```python
from build123d import *

# Parameters (mm, degrees)
SKETCH1_W                    = 31.75
SKETCH1_H                    = 63.5
SKETCH1_W_2                  = 25.4
SKETCH1_H_2                  = 57.15
BOSS_EXTRUDE1_DEPTH          = 685.8
CUT_EXTRUDE1_REACH           = 691.238
SKETCH3_W                    = 50.8
SKETCH3_H                    = 25.4
F_10_0_1935_DIAMETER_HOLE1_D = 4.9149
CUT_EXTRUDE2_REACH           = 691.238
SKETCH6_R                    = 15.5575
SKETCH6_R_2                  = 3.175
CUT_EXTRUDE3_REACH           = 691.238
SKETCH7_R                    = 6.35


with BuildPart() as part:
    # Sketch1 → Boss-Extrude1 (new body)
    with BuildSketch(Plane.XY):
        with Locations((3.710272719, -29.23968021)):
            Rectangle(SKETCH1_W, SKETCH1_H)
        with Locations((3.710272719, -29.23968021)):
            Rectangle(SKETCH1_W_2, SKETCH1_H_2, mode=Mode.SUBTRACT)
    extrude(amount=BOSS_EXTRUDE1_DEPTH)

    # Cut-Extrude1: up to this face of the body (flat: up to its plane)
    cut_extrude1_end = Plane(part.part.faces().sort_by_distance((19.585272719, -29.23968021, 342.9))[0])
    # Sketch3 → Cut-Extrude1 (cut, up to the picked face)
    with BuildSketch(Plane.ZY.offset(12.164727281), mode=Mode.PRIVATE) as cut_extrude1_sk1:
        with BuildLine():
            Line((31.7754, -13.36468021), (120.6754, -13.36468021))
            ThreePointArc((120.6754, -13.36468021), (122.92046403, -14.294616179), (123.8504, -16.53968021))
            Line((123.8504, -16.53968021), (123.8504, -41.93968021))
            ThreePointArc((123.8504, -41.93968021), (122.92046403, -44.18474424), (120.6754, -45.11468021))
            Line((120.6754, -45.11468021), (31.7754, -45.11468021))
            ThreePointArc((31.7754, -45.11468021), (29.53033597, -44.18474424), (28.6004, -41.93968021))
            Line((28.6004, -41.93968021), (28.6004, -16.53968021))
            ThreePointArc((28.6004, -16.53968021), (29.53033597, -14.294616179), (31.7754, -13.36468021))
        make_face()
    cut_extrude1_tool1 = split(extrude(cut_extrude1_sk1.sketch, amount=-CUT_EXTRUDE1_REACH, mode=Mode.PRIVATE), bisect_by=cut_extrude1_end, keep=Keep.BOTH, mode=Mode.PRIVATE)
    # Sketch3 → Cut-Extrude1 (cut, up to the picked face)
    with BuildSketch(Plane.ZY.offset(12.164727281), mode=Mode.PRIVATE) as cut_extrude1_sk2:
        with BuildLine():
            ThreePointArc((657.1996, -41.93968021), (656.26966403, -44.18474424), (654.0246, -45.11468021))
            Line((654.0246, -45.11468021), (565.1246, -45.11468021))
            ThreePointArc((565.1246, -45.11468021), (562.87953597, -44.18474424), (561.9496, -41.93968021))
            Line((561.9496, -41.93968021), (561.9496, -16.53968021))
            ThreePointArc((561.9496, -16.53968021), (562.87953597, -14.294616179), (565.1246, -13.36468021))
            Line((565.1246, -13.36468021), (654.0246, -13.36468021))
            ThreePointArc((654.0246, -13.36468021), (656.26966403, -14.294616179), (657.1996, -16.53968021))
            Line((657.1996, -16.53968021), (657.1996, -41.93968021))
        make_face()
    cut_extrude1_tool2 = split(extrude(cut_extrude1_sk2.sketch, amount=-CUT_EXTRUDE1_REACH, mode=Mode.PRIVATE), bisect_by=cut_extrude1_end, keep=Keep.BOTH, mode=Mode.PRIVATE)
    # Sketch3 → Cut-Extrude1 (cut, up to the picked face)
    with BuildSketch(Plane.ZY.offset(12.164727281), mode=Mode.PRIVATE) as cut_extrude1_sk3:
        with Locations((215.9, -48.28968021)):
            Rectangle(SKETCH3_W, SKETCH3_H)
    cut_extrude1_tool3 = split(extrude(cut_extrude1_sk3.sketch, amount=-CUT_EXTRUDE1_REACH, mode=Mode.PRIVATE), bisect_by=cut_extrude1_end, keep=Keep.BOTH, mode=Mode.PRIVATE)
    # Sketch3 → Cut-Extrude1 (cut, up to the picked face)
    with BuildSketch(Plane.ZY.offset(12.164727281), mode=Mode.PRIVATE) as cut_extrude1_sk4:
        with Locations((469.9, -48.28968021)):
            Rectangle(SKETCH3_W, SKETCH3_H)
    cut_extrude1_tool4 = split(extrude(cut_extrude1_sk4.sketch, amount=-CUT_EXTRUDE1_REACH, mode=Mode.PRIVATE), bisect_by=cut_extrude1_end, keep=Keep.BOTH, mode=Mode.PRIVATE)
    add(cut_extrude1_tool1.solids().sort_by(Axis((-12.164727, -29.23968, 76.2254), (1, 0, 0)))[0], mode=Mode.SUBTRACT)
    add(cut_extrude1_tool2.solids().sort_by(Axis((-12.164727, -29.23968, 609.5746), (1, 0, 0)))[0], mode=Mode.SUBTRACT)
    add(cut_extrude1_tool3.solids().sort_by(Axis((-12.164727, -48.28968, 215.9), (1, 0, 0)))[0], mode=Mode.SUBTRACT)
    add(cut_extrude1_tool4.solids().sort_by(Axis((-12.164727, -48.28968, 469.9), (1, 0, 0)))[0], mode=Mode.SUBTRACT)

    # #10 (0.1935) Diameter Hole1 (through all)
    with Locations(Plane(origin=(3.710272719, 2.51031979, 677.8625), x_dir=(1, 0, 0), z_dir=(0, 1, 0))):
        with Locations((0, 0), (0, 669.925)):
            Hole(F_10_0_1935_DIAMETER_HOLE1_D / 2)

    # Cut-Extrude2: up to this face of the body (flat: up to its plane)
    cut_extrude2_end = Plane(part.part.faces().sort_by_distance((-12.164727281, -27.832525424, 342.9))[0])
    # Sketch6 → Cut-Extrude2 (cut, up to the picked face)
    with BuildSketch(Plane(origin=(19.585272719, 0, 0), x_dir=(0, 0, -1), z_dir=(1, 0, 0)), mode=Mode.PRIVATE) as cut_extrude2_sk1:
        with Locations(Location((-342.9, -34.00218021, 0), (0, 0, 90))):
            Circle(SKETCH6_R)
    cut_extrude2_tool1 = split(extrude(cut_extrude2_sk1.sketch, amount=-CUT_EXTRUDE2_REACH, mode=Mode.PRIVATE), bisect_by=cut_extrude2_end, keep=Keep.BOTH, mode=Mode.PRIVATE)
    # Sketch6 → Cut-Extrude2 (cut, up to the picked face)
    with BuildSketch(Plane(origin=(19.585272719, 0, 0), x_dir=(0, 0, -1), z_dir=(1, 0, 0)), mode=Mode.PRIVATE) as cut_extrude2_sk2:
        with Locations(Location((-393.7, -34.00218021, 0), (0, 0, 90))):
            Circle(SKETCH6_R)
    cut_extrude2_tool2 = split(extrude(cut_extrude2_sk2.sketch, amount=-CUT_EXTRUDE2_REACH, mode=Mode.PRIVATE), bisect_by=cut_extrude2_end, keep=Keep.BOTH, mode=Mode.PRIVATE)
    # Sketch6 → Cut-Extrude2 (cut, up to the picked face)
    with BuildSketch(Plane(origin=(19.585272719, 0, 0), x_dir=(0, 0, -1), z_dir=(1, 0, 0)), mode=Mode.PRIVATE) as cut_extrude2_sk3:
        with Locations(Location((-434.975, -7.01468021, 0), (0, 0, 90))):
            Circle(SKETCH6_R_2)
    cut_extrude2_tool3 = split(extrude(cut_extrude2_sk3.sketch, amount=-CUT_EXTRUDE2_REACH, mode=Mode.PRIVATE), bisect_by=cut_extrude2_end, keep=Keep.BOTH, mode=Mode.PRIVATE)
    # Sketch6 → Cut-Extrude2 (cut, up to the picked face)
    with BuildSketch(Plane(origin=(19.585272719, 0, 0), x_dir=(0, 0, -1), z_dir=(1, 0, 0)), mode=Mode.PRIVATE) as cut_extrude2_sk4:
        with Locations(Location((-301.625, -7.01468021, 0), (0, 0, 90))):
            Circle(SKETCH6_R_2)
    cut_extrude2_tool4 = split(extrude(cut_extrude2_sk4.sketch, amount=-CUT_EXTRUDE2_REACH, mode=Mode.PRIVATE), bisect_by=cut_extrude2_end, keep=Keep.BOTH, mode=Mode.PRIVATE)
    # Sketch6 → Cut-Extrude2 (cut, up to the picked face)
    with BuildSketch(Plane(origin=(19.585272719, 0, 0), x_dir=(0, 0, -1), z_dir=(1, 0, 0)), mode=Mode.PRIVATE) as cut_extrude2_sk5:
        with Locations(Location((-434.975, -51.46468021, 0), (0, 0, 90))):
            Circle(SKETCH6_R_2)
    cut_extrude2_tool5 = split(extrude(cut_extrude2_sk5.sketch, amount=-CUT_EXTRUDE2_REACH, mode=Mode.PRIVATE), bisect_by=cut_extrude2_end, keep=Keep.BOTH, mode=Mode.PRIVATE)
    # Sketch6 → Cut-Extrude2 (cut, up to the picked face)
    with BuildSketch(Plane(origin=(19.585272719, 0, 0), x_dir=(0, 0, -1), z_dir=(1, 0, 0)), mode=Mode.PRIVATE) as cut_extrude2_sk6:
        with Locations(Location((-301.625, -51.46468021, 0), (0, 0, 90))):
            Circle(SKETCH6_R_2)
    cut_extrude2_tool6 = split(extrude(cut_extrude2_sk6.sketch, amount=-CUT_EXTRUDE2_REACH, mode=Mode.PRIVATE), bisect_by=cut_extrude2_end, keep=Keep.BOTH, mode=Mode.PRIVATE)
    add(cut_extrude2_tool1.solids().sort_by(Axis((19.585273, -34.00218, 342.9), (-1, 0, 0)))[0], mode=Mode.SUBTRACT)
    add(cut_extrude2_tool2.solids().sort_by(Axis((19.585273, -34.00218, 393.7), (-1, 0, 0)))[0], mode=Mode.SUBTRACT)
    add(cut_extrude2_tool3.solids().sort_by(Axis((19.585273, -7.01468, 434.975), (-1, 0, 0)))[0], mode=Mode.SUBTRACT)
    add(cut_extrude2_tool4.solids().sort_by(Axis((19.585273, -7.01468, 301.625), (-1, 0, 0)))[0], mode=Mode.SUBTRACT)
    add(cut_extrude2_tool5.solids().sort_by(Axis((19.585273, -51.46468, 434.975), (-1, 0, 0)))[0], mode=Mode.SUBTRACT)
    add(cut_extrude2_tool6.solids().sort_by(Axis((19.585273, -51.46468, 301.625), (-1, 0, 0)))[0], mode=Mode.SUBTRACT)

    # Sketch7 → Cut-Extrude3 (cut, up to next)
    with BuildSketch(Plane(origin=(19.585272719, 0, 0), x_dir=(0, 0, -1), z_dir=(1, 0, 0)), mode=Mode.PRIVATE) as cut_extrude3_sk1:
        with Locations(Location((-434.975, -7.01468021, 0), (0, 0, 90))):
            Circle(SKETCH7_R)
    cut_extrude3_tool1 = extrude(cut_extrude3_sk1.sketch, amount=-CUT_EXTRUDE3_REACH, mode=Mode.PRIVATE) & part.part
    # Sketch7 → Cut-Extrude3 (cut, up to next)
    with BuildSketch(Plane(origin=(19.585272719, 0, 0), x_dir=(0, 0, -1), z_dir=(1, 0, 0)), mode=Mode.PRIVATE) as cut_extrude3_sk2:
        with Locations(Location((-434.975, -51.46468021, 0), (0, 0, 90))):
            Circle(SKETCH7_R)
    cut_extrude3_tool2 = extrude(cut_extrude3_sk2.sketch, amount=-CUT_EXTRUDE3_REACH, mode=Mode.PRIVATE) & part.part
    # Sketch7 → Cut-Extrude3 (cut, up to next)
    with BuildSketch(Plane(origin=(19.585272719, 0, 0), x_dir=(0, 0, -1), z_dir=(1, 0, 0)), mode=Mode.PRIVATE) as cut_extrude3_sk3:
        with Locations(Location((-301.625, -51.46468021, 0), (0, 0, 90))):
            Circle(SKETCH7_R)
    cut_extrude3_tool3 = extrude(cut_extrude3_sk3.sketch, amount=-CUT_EXTRUDE3_REACH, mode=Mode.PRIVATE) & part.part
    # Sketch7 → Cut-Extrude3 (cut, up to next)
    with BuildSketch(Plane(origin=(19.585272719, 0, 0), x_dir=(0, 0, -1), z_dir=(1, 0, 0)), mode=Mode.PRIVATE) as cut_extrude3_sk4:
        with Locations(Location((-301.625, -7.01468021, 0), (0, 0, 90))):
            Circle(SKETCH7_R)
    cut_extrude3_tool4 = extrude(cut_extrude3_sk4.sketch, amount=-CUT_EXTRUDE3_REACH, mode=Mode.PRIVATE) & part.part
    add(cut_extrude3_tool1.solids().sort_by_distance((19.585273, -7.01468, 434.975))[0], mode=Mode.SUBTRACT)
    add(cut_extrude3_tool2.solids().sort_by_distance((19.585273, -51.46468, 434.975))[0], mode=Mode.SUBTRACT)
    add(cut_extrude3_tool3.solids().sort_by_distance((19.585273, -51.46468, 301.625))[0], mode=Mode.SUBTRACT)
    add(cut_extrude3_tool4.solids().sort_by_distance((19.585273, -7.01468, 301.625))[0], mode=Mode.SUBTRACT)


solid = part.part
```
Input: part model. Units: mm. Frame: model coordinates. A direction names the side the tool comes from. Round coordinates to 2 decimals unless told otherwise and drop trailing zeros. Order: outer loops, then holes, each group sorted by start corner. A loop starts at its lowest first (then second) coordinate and runs counter-clockwise, first axis right, second up. Notation, with made-up numbers: (68.5, -31) - (78.5, -31) arc R23 cw to (78.5, -19) - close; hole circle Ø3 at (23.25, 70.5). An arc over 180 degrees is marked (long way). One line per question, with ' | ' between items. Start each with the question number.
1) Pull-direction query (X, two-part tool) for faces 6 (the flat face through (-12.165, -16, 338)), 7 (the flat face through (4, -57.815, 589)), 8 (the cylindrical face through (18.02, -7.84, 441.27)); classes: +X half, -X half, draft (parallel to the pull), parting line (faces both ways), or undercut.
2) Cut plane A-A, the plane z = 618. Return the cut outline in (x, y).
3) Set-up query: faces 1 (the flat face through (4, -0.665, 338)), 2 (the cylindrical face through (18.02, -19.63, 336.94)), 3 (the flat face through (4, -59, 241.3)), 4 (the flat face through (3, -60.99, 94)), 5 (the cylindrical face through (18.02, -52.29, 307.92)). Return all of +Z, -Z, +X, -X, +Y, -Y with unobstructed straight access to the full face (end or side cutting, diameter ignored); none if empty.
4) Ray query, probe 1 along X at (y, z) = (-37, 256.5); probe 2 along Y at (x, z) = (4.5, 114.5); probe 3 along Y at (x, z) = (4, 452). Return the intervals inside material, ascending.
5) Cut plane C-C, the plane z = 342.9. Return the cut outline in (x, y).
6) Cut plane B-B, the plane z = 266. Return the cut outline in (x, y), then the cut area to 3 significant figures.
7) Contact query for flat-ended pins moving along their axis: P1, Ø4, axis at x = 13.5, y = -51, coming from the -Z side; P2, Ø2.5, axis at x = -10, z = 461, coming from the -Y side; P3, Ø7.5, axis at y = -7.01, z = 434.98, coming from the +X side. Output: stop coordinate, or through.
Worked out:
1) face 6: -X half | face 7: undercut | face 8: draft
2) outline: (-12.16, -60.99) - (19.59, -60.99) - (19.59, -45.11) - (16.41, -45.11) - (16.41, -57.81) - (-8.99, -57.81) - (-8.99, -45.11) - (-12.16, -45.11) - close; (-12.16, -13.36) - (-8.99, -13.36) - (-8.99, -0.66) - (16.41, -0.66) - (16.41, -13.36) - (19.59, -13.36) - (19.59, 2.51) - (-12.16, 2.51) - close
3) face 1: +Z, -Z | face 2: +X, -X | face 3: +X, -X, -Y | face 4: +Z, -Z, +X, -X, -Y | face 5: +X
4) probe 1: x = -12.16 to -8.99, 16.41 to 19.59 | probe 2: y = -60.99 to -57.81, -0.66 to 2.51 | probe 3: y = -0.66 to 2.51
5) outline: (-12.16, -60.99) - (19.59, -60.99) - (19.59, -49.56) - (16.41, -49.56) - (16.41, -57.81) - (-8.99, -57.81) - (-8.99, -49.56) - (-12.16, -49.56) - close; (-12.16, -18.44) - (-8.99, -18.44) - (-8.99, -0.66) - (16.41, -0.66) - (16.41, -18.44) - (19.59, -18.44) - (19.59, 2.51) - (-12.16, 2.51) - close
6) outline: (-12.16, -60.99) - (19.59, -60.99) - (19.59, 2.51) - (-12.16, 2.51) - close; hole (-8.99, -57.81) - (16.41, -57.81) - (16.41, -0.66) - (-8.99, -0.66) - close | area: 565 mm^2
7) P1: passes through | P2: stops at y = -35.59 | P3: stops at x = -8.99
